Study the drawing (mm; zero at the part's minimum x, y, z) and answer. A direction names the side the tool comes from. Give positions to 0.01 mm unless a question says otherwise; leave off trailing zeros. Write each loop counter-clockwise with the first axis right and the second up, starting at its lowest first coordinate (ties: lowest second). Pieces come first, ordered by that corner, then holes. Notation, with made-up numbers: M 57,-19 L 105,-19 A29 ccw 105,5 Z; hole C 84,-5 d10. An arc over 180 degrees is marked long. Use a Markdown table: item, result. Add a question column.
Item 1: A cutting plane is placed at C-C on y = 4. Determine the outline of the cut face in (x, z).
Item 2: A cutting plane is placed at A-A on z = 26.5. Determine the outline of the cut face in (x, y).
Item 3: Consider probe 1 along Z at (x, y) = (0.95, 12.5); probe 2 along Y at (x, z) = (1.9, 24.75); probe 3 along Z at (x, y) = (0.3, 20.75) (1 decimal). Determine where each line is inside the solid, lowest interval first. Write a range as [from, to].
Item 4: For the marked faces 1, 2 and 3, determine the directions among +Z, -Z, +X, -X, +Y, -Y from which every point of the face is accessible in a straight line to the end or side of a thin tool.
Item 5: A cutting plane is placed at B-B on x = 1. Determine the outline of the cut face in (y, z).
Item 6: Given P1, Ø0.6, axis at x = 0.5, z = 25.5, coming from the +Y side; P2, Ø0.6, axis at x = 1, z = 27, coming from the -Y side, each flat-ended and moving along its own axis, determine where each tip first touches the part or whether it passes through.
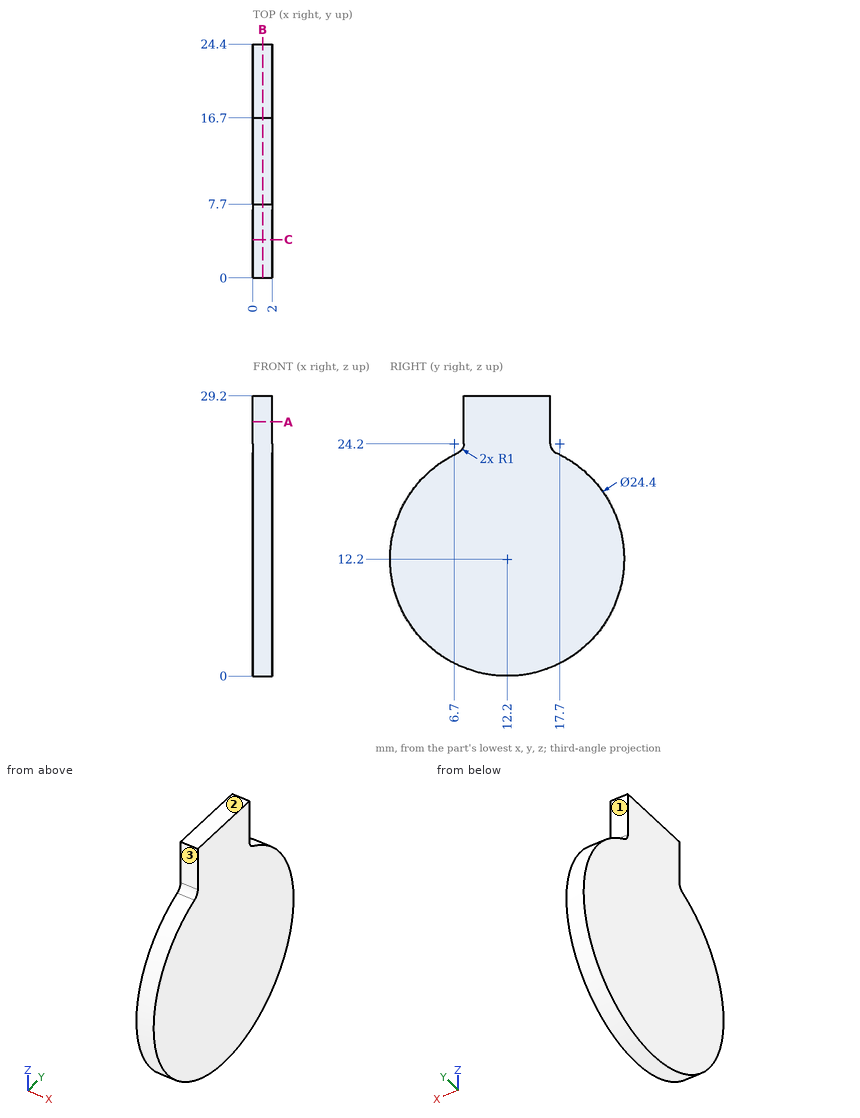
Filled in:
| question | item | result |
|---|---|---|
| 1 | outline | M 0,3.17 L 2,3.17 L 2,21.23 L 0,21.23 Z |
| 2 | outline | M 0,7.7 L 2,7.7 L 2,16.7 L 0,16.7 Z |
| 3 | probe 1 | [0, 29.2] |
| 3 | probe 2 | [7.7, 16.7] |
| 3 | probe 3 | [3.5, 20.9] |
| 4 | face 1 | +Z, +X, -X, +Y |
| 4 | face 2 | +Z, +X, -X, +Y, -Y |
| 4 | face 3 | +Z, +X, -X, -Y |
| 5 | outline | M 7.12,23.29 A12.2 ccw long 17.28,23.29 A1 cw 16.7,24.2 L 16.7,29.2 L 7.7,29.2 L 7.7,24.2 A1 cw Z |
| 6 | P1 | y = 16.7 |
| 6 | P2 | y = 7.7 |
